```python
from build123d import *

# Parameters (mm, degrees)
SKETCH1_W           = 160
SKETCH1_H           = 50
BOSS_EXTRUDE1_DEPTH = 3
SKETCH3_W           = 160
SKETCH3_H           = 1
CUT_EXTRUDE1_DEPTH  = 1.5
SKETCH4_W           = 5
SKETCH4_H           = 65
BOSS_EXTRUDE2_DEPTH = 1.5
SKETCH5_W           = 2
SKETCH5_H           = 65
BOSS_EXTRUDE3_DEPTH = 2
FILLET1_R           = 2
SKETCH8_W           = 160
SKETCH8_H           = 5
BOSS_EXTRUDE4_DEPTH = 2
SKETCH6_W           = 5
SKETCH6_H           = 160
BOSS_EXTRUDE5_DEPTH = 2
SKETCH10_W          = 160
SKETCH10_H          = 3
BOSS_EXTRUDE6_DEPTH = 5
SKETCH13_W          = 10
SKETCH13_H          = 47.007429362
BOSS_EXTRUDE7_DEPTH = 5


with BuildPart() as part:
    # Sketch1 → Boss-Extrude1 (new body)
    with BuildSketch(Plane(origin=(0, 0, 0), x_dir=(0, 0, -1), z_dir=(1, 0, 0))):
        Rectangle(SKETCH1_W, SKETCH1_H)
    extrude(amount=BOSS_EXTRUDE1_DEPTH)

    # Sketch3 → Cut-Extrude1 (cut)
    with BuildSketch(Plane(origin=(3, 0, 0), x_dir=(0, 0, -1), z_dir=(1, 0, 0))):
        with Locations((0, -17.5)):
            Rectangle(SKETCH3_W, SKETCH3_H)
        with Locations((0, -6.5)):
            Rectangle(SKETCH3_W, SKETCH3_H)
        with Locations((0, 4.5)):
            Rectangle(SKETCH3_W, SKETCH3_H)
        with Locations((0, 15.5)):
            Rectangle(SKETCH3_W, SKETCH3_H)
    extrude(amount=-CUT_EXTRUDE1_DEPTH, mode=Mode.SUBTRACT)

    # Sketch4 → Boss-Extrude2 (add, symmetric)
    with BuildSketch(Plane(origin=(3, 0, 0), x_dir=(0, 0, -1), z_dir=(1, 0, 0))):
        with Locations((-37.5, 7.5)):
            Rectangle(SKETCH4_W, SKETCH4_H)
        with Locations((17.5, 7.5)):
            Rectangle(SKETCH4_W, SKETCH4_H)
        with Locations((72.5, 7.5)):
            Rectangle(SKETCH4_W, SKETCH4_H)
    extrude(amount=BOSS_EXTRUDE2_DEPTH, both=True)

    # Sketch5 → Boss-Extrude3 (add)
    with BuildSketch(Plane(origin=(4.5, 0, 0), x_dir=(0, 0, -1), z_dir=(1, 0, 0))):
        with Locations((-39, 7.5)):
            Rectangle(SKETCH5_W, SKETCH5_H)
        with Locations((16, 7.5)):
            Rectangle(SKETCH5_W, SKETCH5_H)
        with Locations((71, 7.5)):
            Rectangle(SKETCH5_W, SKETCH5_H)
    extrude(amount=BOSS_EXTRUDE3_DEPTH)

    # Fillet1
    fillet1_edges = [part.edges().sort_by_distance(p)[0] for p in [
        (6.5, 40, -71),
        (6.5, 40, -16),
        (6.5, 40, 39),
    ]]
    fillet(fillet1_edges, radius=FILLET1_R)

    # Sketch8 → Boss-Extrude4 (add)
    with BuildSketch(Plane.ZY):
        with Locations((0, 29.5)):
            Rectangle(SKETCH8_W, SKETCH8_H)
        with Locations((0, 37.5)):
            Rectangle(SKETCH8_W, SKETCH8_H)
    extrude(amount=-BOSS_EXTRUDE4_DEPTH)

    # Sketch6 → Boss-Extrude5 (add)
    with BuildSketch(Plane(origin=(0, 40, 0), x_dir=(1, 0, 0), z_dir=(0, 1, 0))):
        with Locations((2.5, 0)):
            Rectangle(SKETCH6_W, SKETCH6_H)
    extrude(amount=BOSS_EXTRUDE5_DEPTH)

    # Sketch10 → Boss-Extrude6 (add)
    with BuildSketch(Plane.ZY):
        with Locations((0, -23.5)):
            Rectangle(SKETCH10_W, SKETCH10_H)
    extrude(amount=BOSS_EXTRUDE6_DEPTH)

    # Sketch13 → Boss-Extrude7 (add)
    with BuildSketch(Plane.ZY):
        with Locations((-80, 1.496285319)):
            Rectangle(SKETCH13_W, SKETCH13_H)
    extrude(amount=BOSS_EXTRUDE7_DEPTH)


solid = part.part
```
Design review of the part built by this model. Coordinates are the model's own, in mm. A direction names the side the tool comes from. Coordinates: 2 decimals unless noted, no trailing zeros. Order: outer loops, then holes, each group sorted by start corner. A loop starts at its lowest first (then second) coordinate and runs counter-clockwise, first axis right, second up. Notation, with made-up numbers: (79.25, -0.5) - (118.25, -0.5) arc R22 cw to (118.25, 37.5) - close; hole circle Ø6 at (48, 14). An arc over 180 degrees is marked (long way). One line per question, with ' | ' between items.
Q1. The part is to be moulded in two halves that separate along Y. For faces 1 (the flat face through (-2, -22, 1)), 2 (the flat face through (3, -21, -45)), 3 (the flat face through (3, 40, 17)), say which applies: +Y half, -Y half, draft (parallel to the pull), parting line (faces both ways), or undercut.
Answer key:
face 1: +Y half | face 2: draft | face 3: undercut
Q2. Consider section B-B, the plane x = -3.5. Give the boundary of the cut face in (y, z).
Answer key:
outline: (-25, -80) - (-22.01, -80) - (-22.01, -85) - (25, -85) - (25, -75) - (-22, -75) - (-22, 80) - (-25, 80) - close
Q3. To check wall thickness, follow line 1 along Z through (x, y) = (3.25, -1.5); line 2 along Y through (x, z) = (2.25, 20); line 3 along Y through (x, z) = (0.25, -74). State the ranges of each line that lie inside material, in increasing order.
Answer key:
line 1: z = -75 to -70, -20 to -15, 35 to 40 | line 2: y = -25 to -18, -17 to -7, -6 to 4, 5 to 15, 16 to 25, 40 to 42 | line 3: y = -25 to 25, 27 to 32, 35 to 42
Q4. Consider section C-C, the plane y = 22.5. Give the boundary of the cut face in (x, z), then the cut area to 4 significant figures.
Answer key:
outline: (-5, -85) - (0, -85) - (0, -80) - (3, -80) - (3, -75) - (4.5, -75) - (4.5, -72) - (6.5, -72) - (6.5, -70) - (3, -70) - (3, -20) - (4.5, -20) - (4.5, -17) - (6.5, -17) - (6.5, -15) - (3, -15) - (3, 35) - (4.5, 35) - (4.5, 38) - (6.5, 38) - (6.5, 40) - (3, 40) - (3, 80) - (0, 80) - (0, -75) - (-5, -75) - close | area: 564.5 mm2
Q5. Consider section A-A, the plane z = -49. Give the number of separate pieces and of enclosed holes in the cut face, then the cut area to 3 significant figures.
Answer key:
separate pieces: 3 | enclosed holes: 0 | area: 189 mm2
Q6. For faces 4 (the flat face through (2, 30, 60)), 5 (the flat face through (1.5, 34, 38)), 6 (the flat face through (3, -12, -77)), list the 3-axis set-ups (+Z, -Z, +X, -X, +Y, -Y) from which the entire face can be reached by the end or side of a thin tool; tool diameter is ignored.
Answer key:
face 4: +Z, +X | face 5: +Z, -Z, -X | face 6: -Z, +X, -Y
Q7. Clearance check with flat-ended pins moving along their axes: pin 1 Ø0.6 at (x, y) = (5.5, 7.5) entering from -Z; pin 2 Ø2 at (x, z) = (5.5, -28.5) entering from -Y; pin 3 Ø5.5 at (y, z) = (-21, 0.5) entering from +X. State where each tip first meets the part, or that it passes through.
Answer key:
pin 1: stops at z = -72 | pin 2: stops at y = 40 | pin 3: stops at x = 3
